For this review, take the finished solid that the model builds, in its own axes (mm). Face numbers are marked on the shaded views. A direction names the side the tool comes from. Coordinates: 2 decimals unless noted, no trailing zeros. Order: outer loops, then holes, each group sorted by start corner. A loop starts at its lowest first (then second) coordinate and runs counter-clockwise, first axis right, second up.
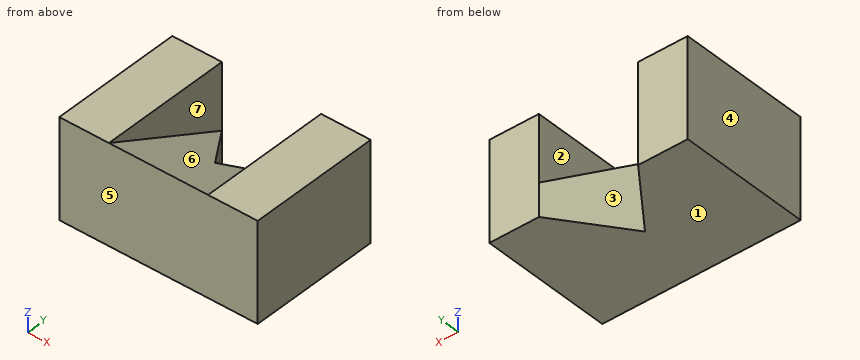
from build123d import *

# Parameters (mm, degrees)
SKETCH_1_W          = 60
SKETCH_1_H          = 30
EXTRUDE_1_DEPTH     = 40
CUT_EXTRUDE_1_DEPTH = 59.309518948
CUT_EXTRUDE_2_DEPTH = 15


with BuildPart() as part:
    # 草圖1 → 填料-伸長1 (new body)
    with BuildSketch(Plane(origin=(0, 0, 0), x_dir=(1, 0, 0), z_dir=(0, 1, 0))):
        with Locations((0, 15)):
            Rectangle(SKETCH_1_W, SKETCH_1_H)
    extrude(amount=EXTRUDE_1_DEPTH)

    # 草圖3 → 除料-伸長1 (cut, through all)
    with BuildSketch(Plane.XY):
        Polygon((-15, 40), (0, 20), (15, 40), align=None)
    extrude(amount=-CUT_EXTRUDE_1_DEPTH, mode=Mode.SUBTRACT)

    # 草圖4 → 除料-伸長2 (cut, symmetric)
    with BuildSketch(Plane(origin=(0, 0, 0), x_dir=(0, 0, -1), z_dir=(1, 0, 0))):
        Polygon((0, 40), (20, 40), (0, 0), align=None)
    extrude(amount=CUT_EXTRUDE_2_DEPTH, both=True, mode=Mode.SUBTRACT)


solid = part.part
1. Take a section at D-D, the plane x = 12. Give the boundary of the cut face in (y, z), plus the area to 3 significant figures.
Answer below:
outline: (0, -30) - (36, -30) - (36, -18) - (0, 0) - close
area: 756 mm2
2. To check wall thickness, follow L1, parallel to X at y = 29.5, z = -8; L2, parallel to X at y = 33.5, z = -20.5 (3 decimals); L3, parallel to Z at x = -10, y = 26. State the ranges of each line that lie inside material, in increasing order.
Answer below:
L1: x = -30 to -15, 15 to 30
L2: x = -30 to -10.125, 10.125 to 30
L3: z = -30 to -13
3. Clearance check with a flat-ended pin moving along its axis: pin 1 Ø1.5 at (x, z) = (-6.5, -3.5) entering from +Y. State where the tip first meets the part, or that it passes through.
Answer below:
pin 1: stops at y = 8.5
4. Take a section at B-B, the plane y = 13. Give the boundary of the cut face in (x, z).
Answer below:
outline: (-30, -30) - (30, -30) - (30, 0) - (15, 0) - (15, -6.5) - (-15, -6.5) - (-15, 0) - (-30, 0) - close
5. The part is to be moulded in two halves that separate along X. For the marked faces 4, 5, 6 and 7, say which applies: +X half, -X half, draft (parallel to the pull), parting line (faces both ways), or undercut.
Answer below:
face 4: -X half
face 5: draft
face 6: undercut
face 7: undercut
6. Take a section at C-C, the plane z = -12. Give the boundary of the cut face in (x, y), plus the area to 3 significant figures.
Answer below:
outline: (-30, 0) - (30, 0) - (30, 40) - (15, 40) - (15, 24) - (3, 24) - (0, 20) - (-3, 24) - (-15, 24) - (-15, 40) - (-30, 40) - close
area: 1,910 mm2
7. Machinability: for the marked faces 1, 2 and 3, which of the approach directions +Z, -Z, +X, -X, +Y, -Y give a long, thin tool a straight path to every point of the face, cutting with its end or side? Answer none if there is none.
Answer below:
face 1: -Z, +X, -X, +Y, -Y
face 2: +Z, +Y
face 3: +Z, -Z, +Y
8. Take a section at A-A, the plane y = 24. Give the boundary of the cut face in (x, z).
Answer below:
outline: (-30, -30) - (-3, -30) - (-3, -12) - (-15, -12) - (-15, 0) - (-30, 0) - close; (3, -30) - (30, -30) - (30, 0) - (15, 0) - (15, -12) - (3, -12) - close
